Here's the drawing with two shaded views (mm, measured from the low corner). I have some questions. A direction names the side the tool comes from. Round coordinates to 2 decimals unless told otherwise and drop trailing zeros. Order: outer loops, then holes, each group sorted by start corner. A loop starts at its lowest first (then second) coordinate and runs counter-clockwise, first axis right, second up. Notation, with made-up numbers: (72.5, -19) -> (122.5, -19) arc R25 cw to (122.5, 19) -> close; hole circle Ø7 at (14, -8). An arc over 180 degrees is marked (long way). Use a Markdown table: item, result. Add a question column.
Q1. If we section it at C-C on y = 55.75: List the corners of the cut face in (x, z) for me, plus the area to 3 significant figures.
Q2. I'm going to push flat-ended pins straight in: pin 1 Ø2.5 at (x, z) = (50.5, 24) entering from +Y; pin 2 Ø14.5 at (x, z) = (31, 9.5) entering from -Y; pin 3 Ø1 at (y, z) = (85, 21.5) entering from -X. Where does each tip first touch, or does it pass through?
Q3. If we section it at A-A on y = 32.5: List the corners of the cut face in (x, z) for me.
Q4. For the marked faces 1, 2 and 3, which set-ups out of +Z, -Z, +X, -X, +Y, -Y let a thin tool reach every point of the face, with its end or its side?
Q5. If we section it at D-D on z = 2: List the corners of the cut face in (x, y) for me, plus the area to 3 significant figures.
Q6. I need wall thicknesses on line 1 along Y through (x, z) = (73.05, 23.75); line 2 along Z through (x, y) = (73, 75.5); line 3 along Y through (x, z) = (49, 12). Which ranges of each line are inside material? Lowest first, please. Write a range as [from, to].
Q7. If we section it at B-B on x = 73.05: List the corners of the cut face in (y, z) for me.
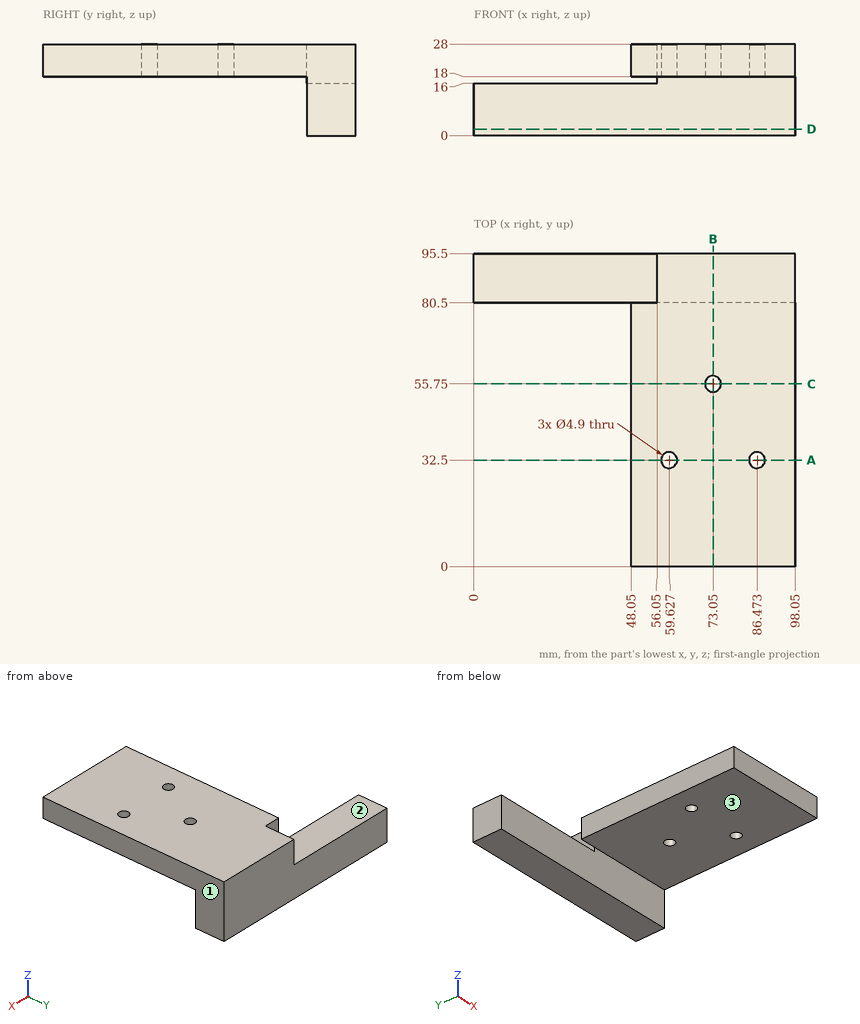
Answer below:
| question | item | result |
|---|---|---|
| 1 | outline | (48.05, 18) -> (70.6, 18) -> (70.6, 28) -> (48.05, 28) -> close; (75.5, 18) -> (98.05, 18) -> (98.05, 28) -> (75.5, 28) -> close |
| 1 | area | 451 mm² |
| 2 | pin 1 | y = 80.5 |
| 2 | pin 2 | y = 80.5 |
| 2 | pin 3 | x = 56.05 |
| 3 | outline | (48.05, 18) -> (57.18, 18) -> (57.18, 28) -> (48.05, 28) -> close; (62.08, 18) -> (84.02, 18) -> (84.02, 28) -> (62.08, 28) -> close; (88.92, 18) -> (98.05, 18) -> (98.05, 28) -> (88.92, 28) -> close |
| 4 | face 1 | +Z, -Z, +X, +Y, -Y |
| 4 | face 2 | +Z, -X, +Y, -Y |
| 4 | face 3 | -Z, +X, -X, -Y |
| 5 | outline | (0, 80.5) -> (98.05, 80.5) -> (98.05, 95.5) -> (0, 95.5) -> close |
| 5 | area | 1,470 mm² |
| 6 | line 1 | [0, 53.3], [58.2, 95.5] |
| 6 | line 2 | [18, 28] |
| 6 | line 3 | [80.5, 95.5] |
| 7 | outline | (0, 18) -> (53.3, 18) -> (53.3, 28) -> (0, 28) -> close; (58.2, 18) -> (80.5, 18) -> (80.5, 0) -> (95.5, 0) -> (95.5, 28) -> (58.2, 28) -> close |
